```python
from build123d import *

# Parameters (mm, degrees)
SKETCH_W        = 11.699997
SKETCH_H        = 32.48951
PAD_DEPTH       = 10.966
SKETCH001_R     = 4.070736
POCKET_DEPTH    = 56
SKETCH002_R     = 1.75554
SKETCH002_R_2   = 1.74777
POCKET001_DEPTH = 71
SKETCH003_R     = 2.5
POCKET002_DEPTH = 5


with BuildPart() as part:
    # Sketch → Pad (new body)
    with BuildSketch(Plane.YZ.offset(-28.95)):
        with Locations((-5.855995, -66.44524)):
            Rectangle(SKETCH_W, SKETCH_H)
    extrude(amount=PAD_DEPTH)

    # Sketch001 (on Face1 of Pad) → Pocket (cut)
    with BuildSketch(Plane(origin=(0, -11.705994, 0), x_dir=(0, 0, -1), z_dir=(0, -1, 0))):
        with Locations((63.03607, -28.441665)):
            Circle(SKETCH001_R)
    extrude(amount=-POCKET_DEPTH, mode=Mode.SUBTRACT)

    # Sketch002 (on Face5 of Pocket) → Pocket001 (cut)
    with BuildSketch(Plane.YZ.offset(-17.984)):
        with Locations((-5.869027, -54.605738)):
            Circle(SKETCH002_R)
        with Locations((-5.877423, -74.910813)):
            Circle(SKETCH002_R_2)
    extrude(amount=-POCKET001_DEPTH, mode=Mode.SUBTRACT)

    # Sketch003 (on Face6 of Pocket001) → Pocket002 (cut)
    with BuildSketch(Plane.YZ.offset(-17.984)):
        with Locations((-5.873042, -54.603773)):
            Circle(SKETCH003_R)
        with Locations((-5.897727, -74.902628)):
            Circle(SKETCH003_R)
    extrude(amount=-POCKET002_DEPTH, mode=Mode.SUBTRACT)


with BuildPart() as part_1:
    # Body placement: moved
    add(part.part.moved(Location((0, 162, 0))))


solid = part_1.part
```
Geometry: final body of the model. Coordinates: model frame, mm. A direction names the side the tool comes from. Round coordinates to 2 decimals unless told otherwise and drop trailing zeros. Write each loop counter-clockwise with the first axis right and the second up, starting at its lowest first coordinate (ties: lowest second). Pieces come first, ordered by that corner, then holes. Notation, with made-up numbers: M 69,-32.75 L 94,-32.75 A22 ccw 94,-20.75 Z; hole C 25,34.25 d9. An arc over 180 degrees is marked long. Answer in a Markdown table with one row per item. Add a question column.
(1) Cut plane C-C, the plane z = -55. Return the cut outline in (x, y), then the cut area to 3 significant figures.
(2) Ray query, L1, parallel to Z at x = -20.5, y = 156; L2, parallel to Y at x = -21.75, z = -75; L3, parallel to Z at x = -28.25, y = 153.25. Return the intervals inside material, ascending.
(3) Contact query for flat-ended pins moving along their axis: pin 1 (3 mm diameter, centred on y = 156.12, z = -74.91, fed in from +X); pin 2 (4.5 mm diameter, centred on y = 156.13, z = -54.6, fed in from +X). Output: stop coordinate, or through.
(4) Draft query along Z for faces 1 (the face through (-24, 156, -50.2)), 2 (the face through (-24.372, 156.062, -63.133)), 3 (the face through (-28.95, 156, -73)). Return one class per face: pulls with the +Z half, pulls with the -Z half, needs draft (parallel to the pull), parting line crosses it, or undercut.
(5) Reachability of faces 4 (the face through (-22.984, 154, -55)), 5 (the face through (-17.984, 156, -66)) from +Z, -Z, +X, -X, +Y, -Y: full face, straight path, thin tool, end or side. Return the list, or none.
(6) Cut plane B-B, the plane x = -27. Return the cut outline in (y, z), then the cut area to 3 significant figures.
(7) Cut plane D-D, the plane y = 160. Return the cut outline in (x, z), then the cut area to 3 significant figures.
(8) Cut plane A-A, the plane y = 155.75. Return the cut outline in (x, z), then the cut area to 3 significant figures.
Established:
| question | item | result |
|---|---|---|
| 1 | outline | M -28.95,150.29 L -17.98,150.29 L -17.98,153.66 L -22.98,153.66 L -22.98,154.42 L -28.95,154.42 Z; M -28.95,157.84 L -22.98,157.84 L -22.98,158.6 L -17.98,158.6 L -17.98,161.99 L -28.95,161.99 Z |
| 1 | area | 83.2 mm² |
| 2 | L1 | -82.69 to -77.4, -72.4 to -57.1, -52.11 to -50.2 |
| 2 | L2 | 150.29 to 153.6, 158.6 to 161.99 |
| 2 | L3 | -82.69 to -67.1, -58.97 to -50.2 |
| 3 | pin 1 | through |
| 3 | pin 2 | x = -22.98 |
| 4 | face 1 | pulls with the +Z half |
| 4 | face 2 | undercut |
| 4 | face 3 | needs draft |
| 5 | face 4 | +X |
| 5 | face 5 | +Z, -Z, +X, +Y, -Y |
| 6 | outline | M 150.29,-82.69 L 161.99,-82.69 L 161.99,-66.84 L 150.29,-66.84 Z; M 150.29,-59.23 L 161.99,-59.23 L 161.99,-50.2 L 150.29,-50.2 Z; hole C 156.12,-74.91 d3.5; hole C 156.13,-54.61 d3.51 |
| 6 | area | 272 mm² |
| 7 | outline | M -28.95,-82.69 L -17.98,-82.69 L -17.98,-50.2 L -28.95,-50.2 L -28.95,-59 A4.07 cw long -28.95,-67.07 Z |
| 7 | area | 326 mm² |
| 8 | outline | M -28.95,-82.69 L -17.98,-82.69 L -17.98,-77.38 L -22.98,-77.38 L -22.98,-76.62 L -28.95,-76.62 Z; M -28.95,-73.2 L -22.98,-73.2 L -22.98,-72.43 L -17.98,-72.43 L -17.98,-57.08 L -22.98,-57.08 L -22.98,-56.32 L -28.95,-56.32 L -28.95,-59 A4.07 cw long -28.95,-67.07 Z; M -28.95,-52.89 L -22.98,-52.89 L -22.98,-52.13 L -17.98,-52.13 L -17.98,-50.2 L -28.95,-50.2 Z |
| 8 | area | 236 mm² |
